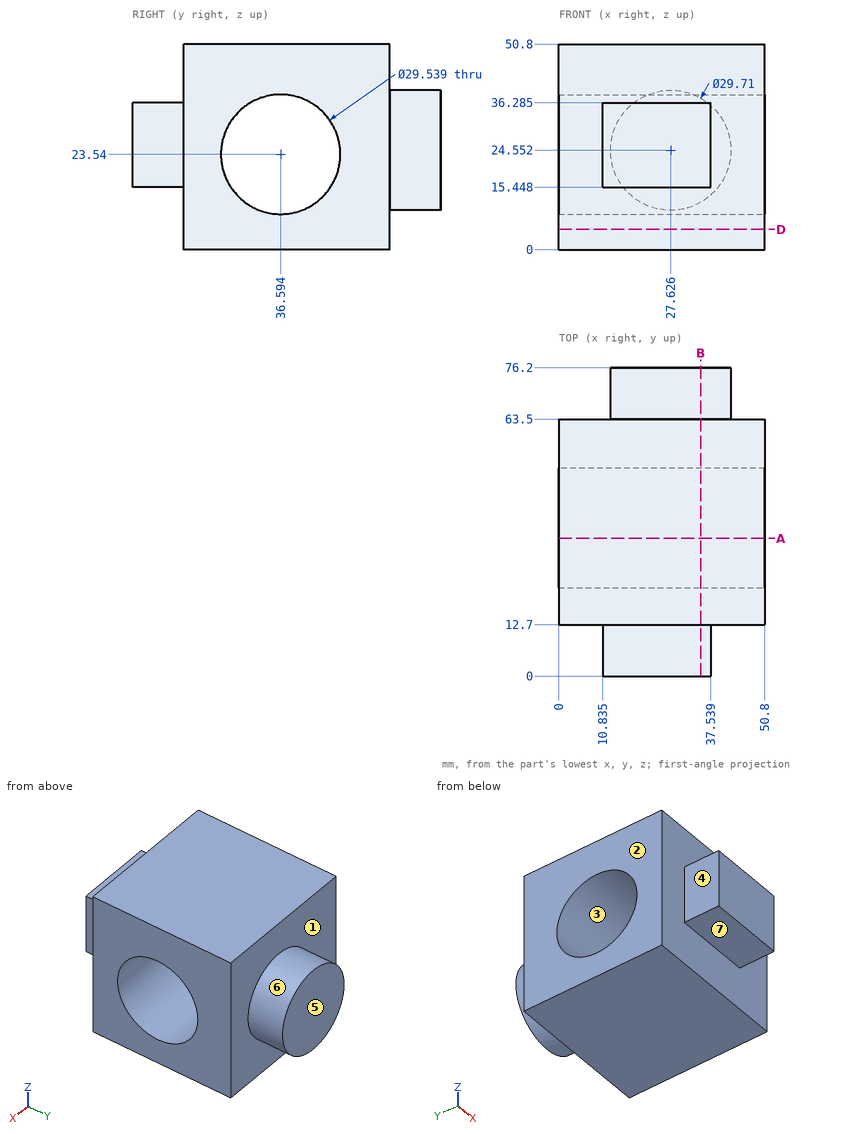
Geometry check sheet. Reference: drawing and pictorial views, mm from the part's lowest x, y, z. A direction names the side the tool comes from. Round coordinates to 2 decimals unless told otherwise and drop trailing zeros. Write each loop counter-clockwise with the first axis right and the second up, starting at its lowest first coordinate (ties: lowest second). Pieces come first, ordered by that corner, then holes. Notation, with made-up numbers: (59, 36.25) -> (69, 36.25) arc R14 ccw to (69, 48.25) -> close; hole circle Ø4 at (13, 83). An arc over 180 degrees is marked (long way). Answer as CSV lines item,"result". Start each with the question number.
1) Section check A-A on y = 34. Enter the section's corners in (x, z), and give its area (3 significant figures).
2) Tool access check on the marked faces 4, 5, 6 and 7. Record the directions out of +Z, -Z, +X, -X, +Y, -Y that give a thin tool (end or side, any length) a straight path to the whole face; none if there is none.
3) Section check B-B on x = 35. Enter the section's corners in (y, z) (1 decimal).
4) Section check D-D on z = 5. Enter the section's corners in (x, y), and give its area (3 significant figures).
5) Go/stop test with flat-tipped pins: P1, Ø1, axis at y = 52.5, z = 11.5, coming from the -X side; P2, Ø10, axis at x = 26.5, y = 6.5, coming from the +Z side (3 decimals); P3, Ø6.5, axis at y = 8, z = 27.5, coming from the -X side (3 decimals). Record where each tip stops, or that it passes through.
6) Material ranges on line 1 (Y direction, x = 20, z = 46); line 2 (Z direction, x = 19.5, y = 25); line 3 (Y direction, x = 19, z = 36) (1 decimal), recorded low to high. Write a range as from..to.
7) Release check for a two-part mould opening along Y. For the marked faces 1, 2 and 3 record: pulls with the +Y half, pulls with the -Y half, needs draft (parallel to the pull), parting line crosses it, or undercut.
Found:
1,outline,"(0, 0) -> (50.8, 0) -> (50.8, 9) -> (0, 9) -> close; (0, 38.08) -> (50.8, 38.08) -> (50.8, 50.8) -> (0, 50.8) -> close"
1,area,"1,100 mm^2"
2,face 4,"+Z, -Z, -X, -Y"
2,face 5,"+Z, -Z, +X, -X, +Y"
2,face 6,"+Y"
2,face 7,"-Z, +X, -X, -Y"
3,outline,"(0, 15.4) -> (12.7, 15.4) -> (12.7, 0) -> (63.5, 0) -> (63.5, 11.7) -> (76.2, 11.7) -> (76.2, 37.4) -> (63.5, 37.4) -> (63.5, 50.8) -> (12.7, 50.8) -> (12.7, 36.3) -> (0, 36.3) -> close; hole circle Ø29.5 at (36.6, 23.5)"
4,outline,"(0, 12.7) -> (50.8, 12.7) -> (50.8, 63.5) -> (0, 63.5) -> close"
4,area,"2,580 mm^2"
5,P1,"stops at x = 0"
5,P2,"stops at z = 36.285"
5,P3,"stops at x = 10.835"
6,line 1,"y = 12.7..63.5"
6,line 2,"z = 0..14.39, 32.69..50.8"
6,line 3,"y = 0..28.7, 44.5..76.2"
7,face 1,"pulls with the +Y half"
7,face 2,"needs draft"
7,face 3,"undercut"
